Can you work these out from the model? Positions are in its coordinate system, mm. Face numbers are marked on the shaded views. Give positions to 0.01 mm unless a question says otherwise; leave off trailing zeros. Loops run counter-clockwise (first coordinate to the right, second up) from the corner with the lowest first, then second, coordinate; pieces in that order, holes last.
from build123d import *

# Parameters (mm, degrees)
F0_W     = 69.863096
F0_H     = 137.526572
F1_DEPTH = 50.8
F2_R     = 9.824635


with BuildPart() as f1:
    # F0 (on Top) → F1 (new body)
    with BuildSketch(Plane.XY):
        with Locations((-34.931548, 0)):
            Rectangle(F0_W, F0_H)
        with Locations((34.931548, 0)):
            Rectangle(F0_W, F0_H)
    extrude(amount=-F1_DEPTH)

    # F4: sweep along a path in F3
    with BuildLine(Plane.XZ) as f4_path:
        ThreePointArc((54.413196, 0), (-0.209475, 53.852413), (-54.832146, 0))
    # F2 (on face) → F4 (sweep)
    with BuildSketch(Plane.XY):
        with Locations((-55.027995, 0.307959)):
            Circle(F2_R)
    sweep(path=f4_path.line)


solid = f1.part
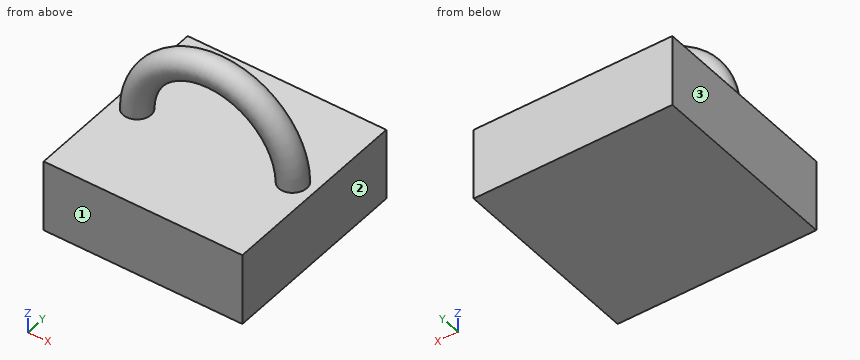
(1) Thinking about a two-plate mould opening in X: for the marked faces 1, 2 and 3, which applies, pulls with the +X half, pulls with the -X half, needs draft (parallel to the pull), parting line crosses it, or undercut?
Returned:
face 1: needs draft
face 2: pulls with the +X half
face 3: pulls with the -X half
(2) Will this pin go through, and if not, where does the flat tip stop? P1, Ø6, axis at x = 23, z = 35.5, coming from the -Y side.
Returned:
P1: stops at y = -4.14
(3) Please list where these lines run through material, in increasing order: probe 1 along Z at (x, y) = (-7, -10.5); probe 2 along Y at (x, z) = (5, 53.5); probe 3 along Y at (x, z) = (-35, 46.5).
Returned:
probe 1: z = -50.8 to 0
probe 2: y = -9.51 to 10.13
probe 3: y = -8.72 to 9.34
(4) Suppose I cut it at A-A on y = -22.5. List the corners of the cut face in (x, z) for me.
Returned:
outline: (-69.86, -50.8) - (69.86, -50.8) - (69.86, 0) - (-69.86, 0) - close
